Input: part model. Units: mm. Frame: model coordinates. A direction names the side the tool comes from. Give positions to 0.01 mm unless a question says otherwise; leave off trailing zeros. Order: outer loops, then holes, each group sorted by start corner. A loop starts at its lowest first (then second) coordinate and runs counter-clockwise, first axis right, second up. Notation, with made-up numbers: (67.25, 39.5) -> (124.25, 39.5) arc R28 cw to (124.25, 74.5) -> close; hole circle Ø1 at (55, 39.25). An arc over 180 degrees is marked (long way). Use a Markdown table: item, result. Add a question column.
from build123d import *

# Parameters (mm, degrees)
SKETCH1_R           = 5.5
SKETCH1_R_2         = 2
BOSS_EXTRUDE1_DEPTH = 5
SKETCH2_R           = 13
CUT_EXTRUDE1_DEPTH  = 2.5
CUT_EXTRUDE2_DEPTH  = 60


with BuildPart() as part:
    # Sketch1 → Boss-Extrude1 (new body)
    with BuildSketch(Plane(origin=(0, 0, 0), x_dir=(1, 0, 0), z_dir=(0, 1, 0))):
        Polygon((7.5, -30), (15, -30), (15, 30), (7.5, 30), (7.5, 35), (-7.5, 35), (-7.5, 30), (-15, 30), (-15, -30), (-7.5, -30), (-7.5, -35), (7.5, -35), align=None)
        with Locations(Location((0, 0, 0), (0, 0, 270))):
            Circle(SKETCH1_R, mode=Mode.SUBTRACT)
        with Locations(Location((0, 8.5, 0), (0, 0, 270))):
            Circle(SKETCH1_R_2, mode=Mode.SUBTRACT)
        with Locations(Location((0, -8.5, 0), (0, 0, 270))):
            Circle(SKETCH1_R_2, mode=Mode.SUBTRACT)
    extrude(amount=BOSS_EXTRUDE1_DEPTH)

    # Sketch2 → Cut-Extrude1 (cut)
    with BuildSketch(Plane(origin=(0, 5, 0), x_dir=(1, 0, 0), z_dir=(0, 1, 0))):
        with Locations(Location((0, 0, 0), (0, 0, 270))):
            Circle(SKETCH2_R)
    extrude(amount=-CUT_EXTRUDE1_DEPTH, mode=Mode.SUBTRACT)

    # Sketch3 → Cut-Extrude2 (cut)
    with BuildSketch(Plane.XY.offset(30)):
        with BuildLine():
            Line((-15, 5), (-15, 2.5))
            ThreePointArc((-15, 2.5), (-14.960745185, 3.752458251), (-14.843134833, 5))
            Line((-14.843134833, 5), (-15, 5))
        make_face()
    extrude(amount=-CUT_EXTRUDE2_DEPTH, mode=Mode.SUBTRACT)


solid = part.part
Q1. Section query B-B (x = 0). Return loops of the section in (y, z).
Q2. Ray query, line 1 (Z direction, x = 0, y = 0.65); line 2 (X direction, y = 1.9, z = 8.5); line 3 (X direction, y = 1.5, z = 0). Return the intervals inside material, ascending.
Q3. Section query A-A (z = 0). Return loops of the section in (x, y), plus the area to 3 significant figures.
Q4. Access query for faces 1 (the flat face through (-7.5, 2, 32)), 2 (the flat face through (11, 2, -30)), 3 (the flat face through (7.5, 2, 33)), 4 (the flat face through (-11, 2, -30)). Directions: +Z, -Z, +X, -X, +Y, -Y. A direction counts if a zero-diameter tool reaches every point of the face in a straight line with its end or side. Return the directions, or none.
Q5. Section query D-D (x = 3.5). Return loops of the section in (y, z).
Q6. Draft query along X for faces 5 (the flat face through (0, 2.5, 6)), 6 (the flat face through (15, 2, 0)), 7 (the flat face through (11, 2, 30)), 8 (the cylindrical face through (-5.37, 1.23, -1.19)). Return one class per face: +X half, -X half, draft (parallel to the pull), parting line (faces both ways), or undercut.
Q7. First-contact query: pin 1 (10 mm diameter, centred on x = 0, z = 0, fed in from +Y); pin 2 (6.5 mm diameter, centred on x = 0, z = 8.5, fed in from -Y); pin 3 (2.5 mm diameter, centred on x = -10.5, y = 2.5, fed in from +Z); pin 4 (2.5 mm diameter, centred on y = 1.5, z = 33, fed in from +X). Flat tips, straight axial feed; report the tip coordinate or a pass-through.
Q8. Section query C-C (y = 1.5). Return loops of the section in (x, z), plus the area to 3 significant figures.
Solution:
| question | item | result |
|---|---|---|
| 1 | outline | (0, -35) -> (5, -35) -> (5, -13) -> (2.5, -13) -> (2.5, -10.5) -> (0, -10.5) -> close; (0, -6.5) -> (2.5, -6.5) -> (2.5, -5.5) -> (0, -5.5) -> close; (0, 5.5) -> (2.5, 5.5) -> (2.5, 6.5) -> (0, 6.5) -> close; (0, 10.5) -> (2.5, 10.5) -> (2.5, 13) -> (5, 13) -> (5, 35) -> (0, 35) -> close |
| 2 | line 1 | z = -35 to -10.5, -6.5 to -5.5, 5.5 to 6.5, 10.5 to 35 |
| 2 | line 2 | x = -15 to -2, 2 to 15 |
| 2 | line 3 | x = -15 to -5.5, 5.5 to 15 |
| 3 | outline | (-15, 0) -> (-5.5, 0) -> (-5.5, 2.5) -> (-13, 2.5) -> (-13, 5) -> (-14.84, 5) arc R20 ccw to (-15, 2.5) -> close; (5.5, 0) -> (15, 0) -> (15, 5) -> (13, 5) -> (13, 2.5) -> (5.5, 2.5) -> close |
| 3 | area | 57.4 mm² |
| 4 | face 1 | +Z, -X, +Y, -Y |
| 4 | face 2 | -Z, +X, +Y, -Y |
| 4 | face 3 | +Z, +X, +Y, -Y |
| 4 | face 4 | -Z, -X, +Y, -Y |
| 5 | outline | (0, -35) -> (5, -35) -> (5, -12.52) -> (2.5, -12.52) -> (2.5, -4.24) -> (0, -4.24) -> close; (0, 4.24) -> (2.5, 4.24) -> (2.5, 12.52) -> (5, 12.52) -> (5, 35) -> (0, 35) -> close |
| 6 | face 5 | undercut |
| 6 | face 6 | +X half |
| 6 | face 7 | draft |
| 6 | face 8 | undercut |
| 7 | pin 1 | passes through |
| 7 | pin 2 | stops at y = 0 |
| 7 | pin 3 | stops at z = 30 |
| 7 | pin 4 | stops at x = 7.5 |
| 8 | outline | (-15, -30) -> (-7.5, -30) -> (-7.5, -35) -> (7.5, -35) -> (7.5, -30) -> (15, -30) -> (15, 30) -> (7.5, 30) -> (7.5, 35) -> (-7.5, 35) -> (-7.5, 30) -> (-15, 30) -> close; hole circle Ø11 at (0, 0); hole circle Ø4 at (0, -8.5); hole circle Ø4 at (0, 8.5) |
| 8 | area | 1,830 mm² |
